Geometry check sheet. Reference: the model listing, model coordinates, mm. Round coordinates to 2 decimals unless told otherwise and drop trailing zeros. Write each loop counter-clockwise with the first axis right and the second up, starting at its lowest first coordinate (ties: lowest second). Pieces come first, ordered by that corner, then holes. Notation, with made-up numbers: M -14.5,63 L 25.5,63 A8 ccw 25.5,68 Z; hole C -7,-6 d8. An arc over 180 degrees is marked long. Use a Markdown table: item, result.
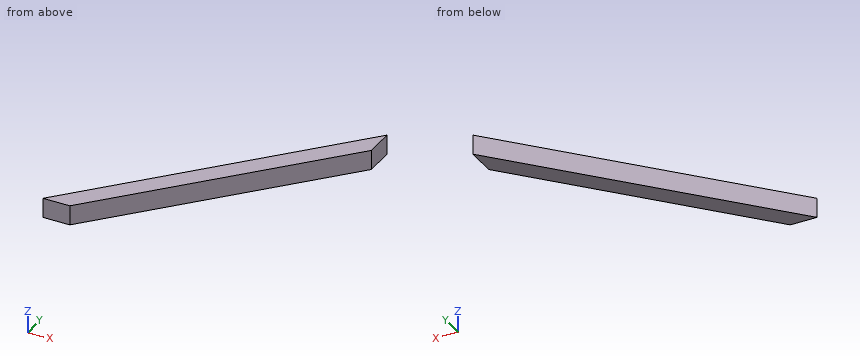
Autodesk Inventor part; units mm, degrees
ref_plane "YZ Plane" through (0, 0, 0) normal (1, 0, 0) x (0, 1, 0)
ref_plane "XZ Plane" through (0, 0, 0) normal (0, 1, 0) x (-1, 0, 0)
ref_plane "XY Plane" through (0, 0, 0) normal (0, 0, 1) x (1, 0, 0)
sketch "Sketch1" plane through (0, 0, 0) normal (0, 0, 1) x (1, 0, 0)
  line L0 (-592.8645, -609.8015) -> (-491.2645, -609.8015)
  line L1 (524.7355, 609.3985) -> (-592.8645, -609.8015)
  line L2 (524.7355, 609.3985) -> (599.6304, 540.7448) construction
  line L3 (524.7355, 459.0414) -> (-455.0371, -609.8015)
  line L4 (-592.8645, -609.8015) -> (-455.0371, -609.8015)
  line L5 (-592.8645, -609.8015) -> (-455.0371, -609.8015)
  line L6 (524.7355, 609.3985) -> (524.7355, 459.0414)
  point P0 (0, 0)
  dimension "d0" = 101.6
extrude "Extrusion1" add sketch "Sketch1" along normal blind 101.6
properties part number "4x4xidkanymore"
Item 1: Material ranges on line 1 along Y through (x, z) = (-365.5, 24); line 2 along Y through (x, z) = (-505.5, 95); line 3 along X through (y, z) = (-179.5, 23), recorded low to high. Write a range as from..to.
Outcome:
| item | result |
|---|---|
| line 1 | y = -512.12..-361.77 |
| line 2 | y = -609.8..-514.49 |
| line 3 | x = -198.42..-60.59 |
Item 2: Cross-section at A-A, the plane z = 57.5. Record the cut outline in (x, y), and give its area (3 significant figures).
Outcome:
| item | result |
|---|---|
| outline | M -592.86,-609.8 L -455.04,-609.8 L 524.74,459.04 L 524.74,609.4 Z |
| area | 158,000 mm2 |
Item 3: Go/stop test with flat-tipped pins: pin 1 (12 mm diameter, centred on y = -191.5, z = 40.5, fed in from +X); pin 2 (5 mm diameter, centred on x = 346, z = 83, fed in from -Y); pin 3 (3 mm diameter, centred on y = -331.5, z = 89.5, fed in from +X). Record where each tip stops, or that it passes through.
Outcome:
| item | result |
|---|---|
| pin 1 | stops at x = -66.09 |
| pin 2 | stops at y = 261.33 |
| pin 3 | stops at x = -198.55 |
Item 4: Cross-section at B-B, the plane x = -327.5. Record the cut outline in (y, z).
Outcome:
| item | result |
|---|---|
| outline | M -470.67,0 L -320.31,0 L -320.31,101.6 L -470.67,101.6 Z |
